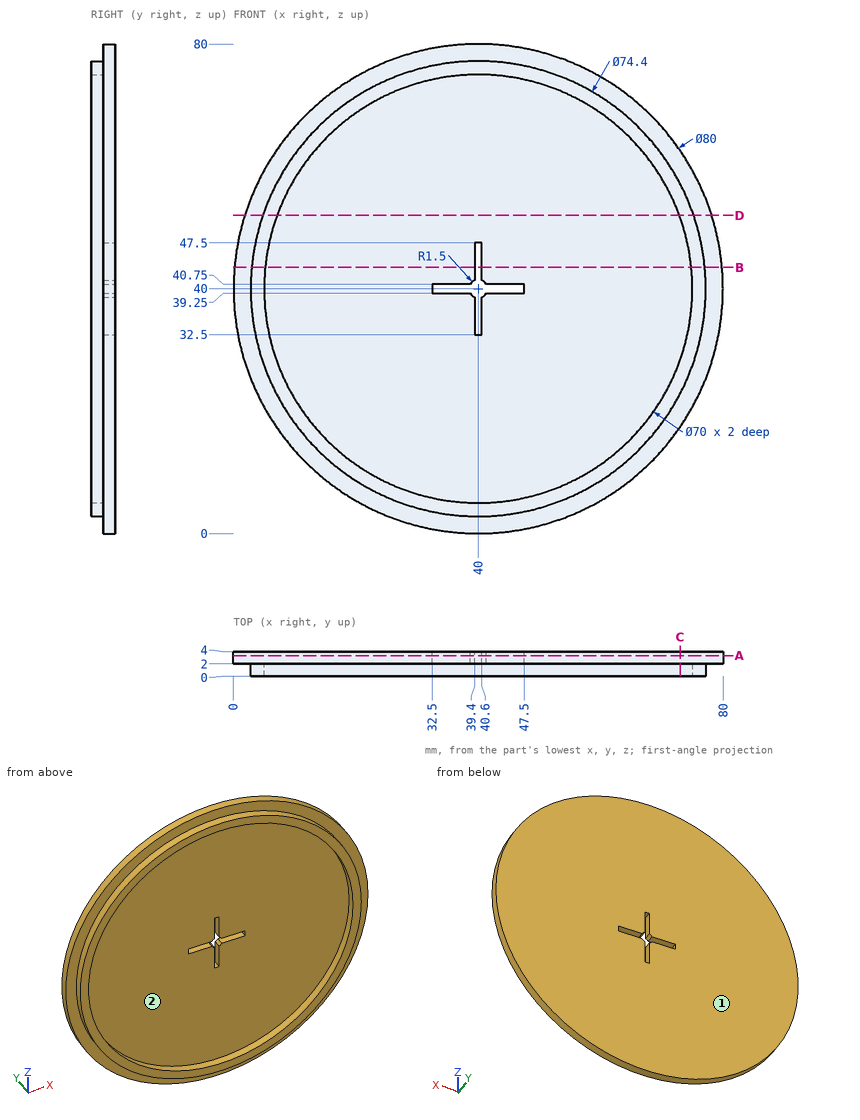
For this review, use the dimensioned drawing (mm, ordinates from the lowest corner) and the shaded views. Give positions to 0.01 mm unless a question says otherwise; leave off trailing zeros. Order: outer loops, then holes, each group sorted by start corner. A loop starts at its lowest first (then second) coordinate and runs counter-clockwise, first axis right, second up.
1. For pin 1 Ø1.6 at (x, y) = (44, 3) entering from -Z; pin 2 Ø1.6 at (y, z) = (3, 44) entering from -X; pin 3 Ø4 at (x, z) = (28.5, 62) entering from -Y, all flat-tipped, find the tip position at first contact; note any pin that passes through.
Solution:
pin 1: stops at z = 0.13
pin 2: stops at x = 0.13
pin 3: stops at y = 2
2. Add section B-B, the plane z = 43.5. State the section outline as (x, y) points (3 decimals), then the cut area to 3 significant figures.
Solution:
outline: (0.153, 2) - (2.965, 2) - (2.965, 0) - (5.175, 0) - (5.175, 2) - (39.4, 2) - (39.4, 4) - (0.153, 4) - close; (40.6, 2) - (74.825, 2) - (74.825, 0) - (77.035, 0) - (77.035, 2) - (79.847, 2) - (79.847, 4) - (40.6, 4) - close
area: 166 mm2
3. Add section A-A, the plane y = 3.35. State the section outline as (x, z) points.
Solution:
outline: circle Ø80 at (40, 40); hole (32.5, 39.25) - (38.7, 39.25) arc R1.5 ccw to (39.4, 38.63) - (39.4, 32.5) - (40.6, 32.5) - (40.6, 38.63) arc R1.5 ccw to (41.3, 39.25) - (47.5, 39.25) - (47.5, 40.75) - (41.3, 40.75) arc R1.5 ccw to (40.6, 41.37) - (40.6, 47.5) - (39.4, 47.5) - (39.4, 41.37) arc R1.5 ccw to (38.7, 40.75) - (32.5, 40.75) - close
4. Add section D-D, the plane z = 52. State the section outline as (x, y) points.
Solution:
outline: (1.84, 2) - (4.79, 2) - (4.79, 0) - (7.12, 0) - (7.12, 2) - (72.88, 2) - (72.88, 0) - (75.21, 0) - (75.21, 2) - (78.16, 2) - (78.16, 4) - (1.84, 4) - close
5. Mouldability with a two-part tool opening along X and no side actions: class the marked faces 1 and 2 as +X half, -X half, draft (parallel to the pull), parting line (faces both ways), or undercut.
Solution:
face 1: draft
face 2: undercut
6. Add section C-C, the plane x = 73. State the section outline as (y, z) points, then the cut area to 3 significant figures.
Solution:
outline: (0, 22.83) - (2, 22.83) - (2, 17.39) - (4, 17.39) - (4, 62.61) - (2, 62.61) - (2, 57.17) - (0, 57.17) - (0, 51.66) - (2, 51.66) - (2, 28.34) - (0, 28.34) - close
area: 112 mm2
7. To check wall thickness, follow L1, parallel to Z at x = 40, y = 0.55; L2, parallel to Y at x = 41.5, z = 25; L3, parallel to Z at x = 19, y = 0.2. State the ranges of each line that lie inside material, in increasing order.
Solution:
L1: z = 2.8 to 5, 75 to 77.2
L2: y = 2 to 4
L3: z = 9.29 to 12, 68 to 70.71
